Read the model definition and answer for the solid it produces. Units are mm, in the model's axes. Face numbers are marked on the shaded views. A direction names the side the tool comes from. Give positions to 0.01 mm unless a question says otherwise; leave off trailing zeros. Write each loop counter-clockwise with the first axis right and the second up, starting at its lowest first coordinate (ties: lowest second). Pieces come first, ordered by that corner, then holes. Notation, with made-up numbers: M 74.5,52.25 L 113.5,52.25 A15 ccw 113.5,81.25 Z; hole C 8.25,-15.75 d10. An arc over 180 degrees is marked long. Use a Markdown table: item, result. Add a question column.
Item 1: Consider probe 1 along X at (y, z) = (-362, 21); probe 2 along Z at (x, y) = (-653.5, -350.75); probe 3 along Y at (x, z) = (-662, 2). Determine where each line is inside the solid, lowest interval first. Write a range as [from, to].
Item 2: A cutting plane is placed at B-B on y = -347.5. Determine the outline of the cut face in (x, z).
Item 3: Given P1, Ø5, axis at x = -668.5, z = 7.5, coming from the +Y side; P2, Ø12, axis at x = -643.5, y = -353, coming from the +Z side; P3, Ø8, axis at x = -622.5, y = -350, coming from the -Z side, each flat-ended and moving along its own axis, determine where each tip first touches the part or whether it passes through.
Item 4: A cutting plane is placed at A-A on z = 18. Determine the outline of the cut face in (x, y).
Item 5: For the marked faces 5, 6, 7, 8 and 9, determine the directions among +Z, -Z, +X, -X, +Y, -Y from which every point of the face is accessible in a straight line to the end or side of a thin tool.
Item 6: A cutting plane is placed at D-D on x = -621.5. Determine the outline of the cut face in (y, z), then the cut area to 3 significant figures.
Item 7: A cutting plane is placed at C-C on z = 31. Determine the outline of the cut face in (x, y).
Item 8: The mould has two halves that part along Y. Classify the marked faces 1, 2, 3 and 4: pulls with the +Y half, pulls with the -Y half, needs draft (parallel to the pull), parting line crosses it, or undercut.
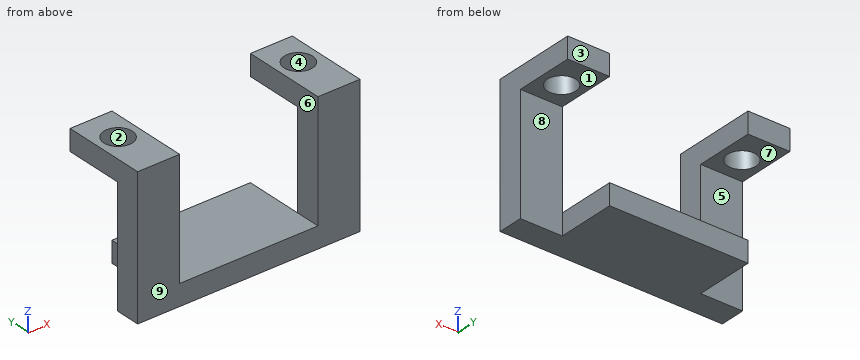
from build123d import *

# Parameters (mm, degrees)
BOSS_EXTRUDE1_DEPTH = 5
SKETCH1_7_W         = 10
SKETCH1_7_H         = 6
BOSS_EXTRUDE2_DEPTH = 33
BOSS_EXTRUDE3_START = 33
SKETCH1_9_W         = 10
SKETCH1_9_H         = 14
SKETCH1_9_R         = 3.4
BOSS_EXTRUDE3_DEPTH = 5


with BuildPart() as part:
    # Sketch1 → Boss-Extrude1 (new body)
    with BuildSketch(Plane.XY):
        Polygon((-628.74225666, -346.426096697), (-661.74225666, -346.426096697), (-661.74225666, -360.426096697), (-661.74225666, -366.426096697), (-628.74225666, -366.426096697), (-628.74225666, -360.426096697), align=None)
    extrude(amount=BOSS_EXTRUDE1_DEPTH)

    # Sketch1<7> → Boss-Extrude2 (add)
    with BuildSketch(Plane.XY):
        with Locations((-623.74225666, -363.426096697)):
            Rectangle(SKETCH1_7_W, SKETCH1_7_H)
        with Locations((-666.74225666, -363.426096697)):
            Rectangle(SKETCH1_7_W, SKETCH1_7_H)
    extrude(amount=BOSS_EXTRUDE2_DEPTH)

    # Sketch1<9> → Boss-Extrude3 (add)
    # profile 1 of 2: a face of its own
    with BuildSketch(Plane.XY.offset(BOSS_EXTRUDE3_START)):
        with Locations((-666.74225666, -353.426096697)):
            Rectangle(SKETCH1_9_W, SKETCH1_9_H)
        with Locations((-666.74225666, -354.426096697)):
            Circle(SKETCH1_9_R, mode=Mode.SUBTRACT)
    # profile 2 of 2: a face of its own
    with BuildSketch(Plane.XY.offset(BOSS_EXTRUDE3_START)):
        with Locations((-623.74225666, -353.426096697)):
            Rectangle(SKETCH1_9_W, SKETCH1_9_H)
        with Locations((-623.74225666, -354.426096697)):
            Circle(SKETCH1_9_R, mode=Mode.SUBTRACT)
    extrude(amount=-BOSS_EXTRUDE3_DEPTH)


solid = part.part
Filled in:
| question | item | result |
|---|---|---|
| 1 | probe 1 | [-671.74, -661.74], [-628.74, -618.74] |
| 1 | probe 2 | [0, 5] |
| 1 | probe 3 | [-366.43, -360.43] |
| 2 | outline | M -671.74,28 L -661.74,28 L -661.74,33 L -671.74,33 Z; M -661.74,0 L -628.74,0 L -628.74,5 L -661.74,5 Z; M -628.74,28 L -618.74,28 L -618.74,33 L -628.74,33 Z |
| 3 | P1 | y = -360.43 |
| 3 | P2 | z = 5 |
| 3 | P3 | z = 28 |
| 4 | outline | M -671.74,-366.43 L -661.74,-366.43 L -661.74,-360.43 L -671.74,-360.43 Z; M -628.74,-366.43 L -618.74,-366.43 L -618.74,-360.43 L -628.74,-360.43 Z |
| 5 | face 5 | -Z, -X, +Y |
| 5 | face 6 | +Z, +Y, -Y |
| 5 | face 7 | -Z, +X, -X, +Y |
| 5 | face 8 | -Z, +X, +Y |
| 5 | face 9 | +Z, -Z, +X, -X, -Y |
| 6 | outline | M -366.43,0 L -360.43,0 L -360.43,28 L -356.98,28 L -356.98,33 L -366.43,33 Z; M -351.87,28 L -346.43,28 L -346.43,33 L -351.87,33 Z |
| 6 | area | 242 mm² |
| 7 | outline | M -671.74,-366.43 L -661.74,-366.43 L -661.74,-346.43 L -671.74,-346.43 Z; M -628.74,-366.43 L -618.74,-366.43 L -618.74,-346.43 L -628.74,-346.43 Z; hole C -666.74,-354.43 d6.8; hole C -623.74,-354.43 d6.8 |
| 8 | face 1 | needs draft |
| 8 | face 2 | undercut |
| 8 | face 3 | pulls with the +Y half |
| 8 | face 4 | undercut |
